The listing builds one solid part. Answer for the finished solid, in the listing's coordinates (mm). Face numbers are marked on the shaded views. A direction names the side the tool comes from. Coordinates: 2 decimals unless noted, no trailing zeros. Order: outer loops, then holes, each group sorted by start corner. A loop starts at its lowest first (then second) coordinate and runs counter-clockwise, first axis right, second up.
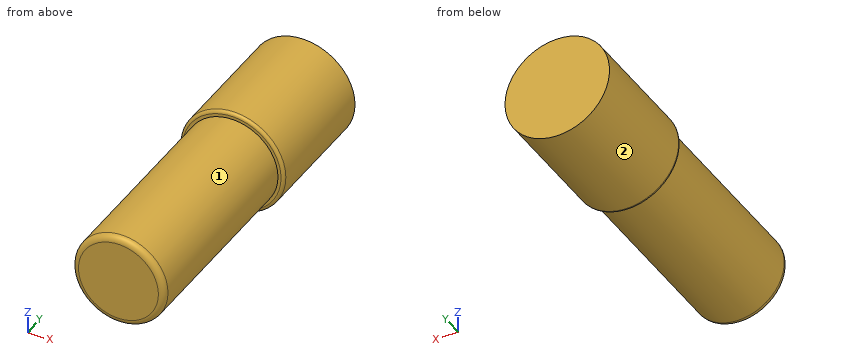
```python
from build123d import *

# Parameters (mm, degrees)
SKETCH011_R  = 3.4
PAD009_DEPTH = 8.25
FILLET004_R  = 0.2
SKETCH012_R  = 3
PAD010_DEPTH = 13.2
FILLET005_R  = 0.4


with BuildPart() as part:
    # Sketch011 → Pad009 (new body)
    with BuildSketch(Plane.XZ):
        Circle(SKETCH011_R)
    extrude(amount=PAD009_DEPTH)

    # Fillet004
    fillet004_edges = [part.edges().sort_by_distance(p)[0] for p in [
        (-3.4, -8.25, 0),
    ]]
    fillet(fillet004_edges, radius=FILLET004_R)

    # Sketch012 (on Face4 of Fillet004) → Pad010 (join)
    with BuildSketch(Plane.XZ.offset(8.25)):
        Circle(SKETCH012_R)
    extrude(amount=PAD010_DEPTH)

    # Fillet005
    fillet005_edges = [part.edges().sort_by_distance(p)[0] for p in [
        (-3, -21.45, 0),
    ]]
    fillet(fillet005_edges, radius=FILLET005_R)


with BuildPart() as part_1:
    # Body019 placement: moved
    add(part.part.moved(Location((0, -1.25, 0))))


solid = part_1.part
```
(1) Each of these flat-tipped pins is pushed along its axis until it touches: pin 1 Ø1.5 at (y, z) = (-8, 2) entering from -X; pin 2 Ø1 at (x, y) = (-1.5, -3.5) entering from +Z. Where does it stop, or does it pass through?
(2) Find section A-A (x = 0). Write down the section's boundary in (y, z), and give its area (3 significant figures).
(3) Consider line 1 (Y direction, x = 2.25, z = -2.25); line 2 (X direction, y = -5.5, z = -3); line 3 (X direction, y = -7.5, z = 0.5). Determine where each line is inside the solid, lowest interval first.
(4) Find section C-C (y = -3). Write down the section's boundary in (x, z), and give its area (3 significant figures).
(5) Find section D-D (y = -19.5). Write down the section's boundary in (x, z).
(6) For the marked faces 1 and 2, determine the directions among +Z, -Z, +X, -X, +Y, -Y from which every point of the face is accessible in a straight line to the end or side of a thin tool.
(7) Find section B-B (z = 0). Write down the section's boundary in (x, y), and give its area (3 significant figures).
Findings below:
1. pin 1: stops at x = -3.16
1. pin 2: stops at z = 3.25
2. outline: (-22.7, -2.6) arc R0.4 ccw to (-22.3, -3) - (-9.5, -3) - (-9.5, -3.2) arc R0.2 ccw to (-9.3, -3.4) - (-1.25, -3.4) - (-1.25, 3.4) - (-9.3, 3.4) arc R0.2 ccw to (-9.5, 3.2) - (-9.5, 3) - (-22.3, 3) arc R0.4 ccw to (-22.7, 2.6) - close
2. area: 135 mm2
3. line 1: y = -9.5 to -1.25
3. line 2: x = -1.6 to 1.6
3. line 3: x = -3.36 to 3.36
4. outline: circle Ø6.8 at (0, 0)
4. area: 36.3 mm2
5. outline: circle Ø6 at (0, 0)
6. face 1: -Y
6. face 2: +Y, -Y
7. outline: (-3.4, -9.3) arc R0.2 ccw to (-3.2, -9.5) - (-3, -9.5) - (-3, -22.3) arc R0.4 ccw to (-2.6, -22.7) - (2.6, -22.7) arc R0.4 ccw to (3, -22.3) - (3, -9.5) - (3.2, -9.5) arc R0.2 ccw to (3.4, -9.3) - (3.4, -1.25) - (-3.4, -1.25) - close
7. area: 135 mm2
